Can you work these out from the model? Positions are in its coordinate system, mm. A direction names the side the tool comes from. Coordinates: 2 decimals unless noted, no trailing zeros. Order: outer loops, then holes, each group sorted by start corner. A loop starts at its lowest first (then second) coordinate and runs counter-clockwise, first axis right, second up.
```python
from build123d import *

# Parameters (mm, degrees)
F0_W      = 3.8989
F0_H      = 3.9624
F1_DEPTH  = 3.175
F3_DEPTH  = 38.1
F5_DEPTH  = 64.262
F7_DEPTH  = 63.5
F9_DEPTH  = 25.4
F10_W     = 76.2
F10_H     = 2.617364
F11_DEPTH = 25.4


with BuildPart() as f1:
    # F0 (on Top) → F1 (new body)
    with BuildSketch(Plane.XY):
        Polygon((38.1, 27.7876), (38.1, 31.75), (-34.2011, 31.75), (-34.2011, 27.7876), (-29.4386, 27.7876), (-21.5011, 27.7876), (-16.7386, 27.7876), (-8.6614, 27.7876), (-3.8989, 27.7876), (-3.884394, 27.7876), (4.0386, 27.7876), (8.789393, 27.7876), (8.8011, 27.7876), (16.7386, 27.7876), (21.459464, 27.7876), (21.5011, 27.7876), (29.4386, 27.7876), (34.2011, 27.7876), (34.226403, 27.7876), align=None)
        with Locations((-36.15055, 29.7688)):
            Rectangle(F0_W, F0_H)
        Polygon((38.1, -31.75), (38.1, 27.7876), (34.226403, 27.7876), (34.226403, 23.0251), (29.4386, 23.0251), (29.4386, 27.7876), (21.5011, 27.7876), (21.459464, 27.7876), (21.459464, 23.0251), (16.7386, 23.0251), (16.7386, 27.7876), (8.8011, 27.7876), (8.789393, 27.7876), (8.789393, 23.0251), (4.0386, 23.0251), (4.0386, 27.7876), (-3.884394, 27.7876), (-3.884394, 23.0251), (-8.6614, 23.0251), (-8.6614, 27.7876), (-16.7386, 27.7876), (-16.7386, 23.0251), (-21.5011, 23.0251), (-21.5011, 27.7876), (-29.4386, 27.7876), (-29.4386, 23.0251), (-34.2011, 23.0251), (-34.2011, 15.0876), (-34.2011, 10.3251), (-34.2011, 2.3876), (-34.2011, -2.3749), (-34.2011, -10.3124), (-34.2011, -15.0749), (-34.2011, -23.0124), (-34.2011, -27.7749), (-34.2011, -31.75), align=None)
        Polygon((-34.2011, 23.0251), (-34.2011, 27.7876), (-38.1, 27.7876), (-38.1, -31.75), (-34.2011, -31.75), (-34.2011, -27.7749), (-34.2011, -23.0124), (-34.2011, -15.0749), (-34.2011, -10.3124), (-34.2011, -2.3749), (-34.2011, 2.3876), (-34.2011, 10.3251), (-34.2011, 15.0876), align=None)
    extrude(amount=F1_DEPTH)

    # F2 (on face) → F3 (join)
    with BuildSketch(Plane.XY.offset(3.175)):
        Polygon((-31.75, -28.575), (-31.75, -31.75), (31.75, -31.75), (31.75, -28.575), (31.75, -25.4), (-31.75, -25.4), align=None)
    extrude(amount=F3_DEPTH)

    # F4 (on face) → F5 (cut)
    with BuildSketch(Plane(origin=(-31.75, 0, 0), x_dir=(0, -1, 0), z_dir=(-1, 0, 0))):
        Polygon((31.75, 41.275), (28.575, 41.275), (31.75, 3.175), align=None)
    extrude(amount=-F5_DEPTH, mode=Mode.SUBTRACT)

    # F6 (on face) → F7 (cut)
    with BuildSketch(Plane.YZ.offset(31.75)):
        Polygon((-31.75, 3.175), (-28.575, 3.175), (-26.9875, 41.275), (-28.575, 41.275), align=None)
    extrude(amount=-F7_DEPTH, mode=Mode.SUBTRACT)

    # F8 (on face) → F9 (cut)
    with BuildSketch(Plane.XY.offset(3.175)):
        Polygon((38.1, -28.575), (-31.75, -28.575), (-38.1, -28.575), (-38.1, -31.75), (38.1, -31.75), align=None)
    extrude(amount=-F9_DEPTH, mode=Mode.SUBTRACT)

    # F10 (on face) → F11 (cut)
    with BuildSketch(Plane.XY.offset(3.175)):
        with Locations((0, 30.441318)):
            Rectangle(F10_W, F10_H)
    extrude(amount=-F11_DEPTH, mode=Mode.SUBTRACT)


solid = f1.part
```
1. On a 3-axis mill with a long thin cutter (end or side, diameter ignored), from which of +Z, -Z, +X, -X, +Y, -Y can I reach the whole of each face in a straight line? I mean faces 5 (the flat face through (-19, 27.788, 2)), 6 (the flat face through (31.75, -27, 22)), 7 (the flat face through (-38.1, 1, 2)). Say none if no direction works.
Completed:
face 5: +Z, -Z
face 6: +Z, +X, +Y, -Y
face 7: +Z, -Z, -X, +Y, -Y
2. Imagine slicing it at A-A on x = 6. Please give me the cut outline in (y, z) (1 decimal).
Completed:
outline: (-28.6, 0) - (23, 0) - (23, 3.2) - (-25.4, 3.2) - (-25.4, 41.3) - (-27, 41.3) - (-28.6, 3.2) - close; (27.8, 0) - (29.1, 0) - (29.1, 3.2) - (27.8, 3.2) - close
3. Imagine slicing it at D-D on z = 15. Please give me the cut outline in (x, y).
Completed:
outline: (-31.75, -28.08) - (31.75, -28.08) - (31.75, -25.4) - (-31.75, -25.4) - close
4. I'm going to push flat-ended pins straight in: pin 1 (1.6 mm diameter, centred on y = -27.5, z = 18.5, fed in from -X); pin 2 (1.5 mm diameter, centred on x = -17.5, y = 11.5, fed in from +Z) (3 decimals). Where does each tip first touch, or does it pass through?
Completed:
pin 1: stops at x = -31.75
pin 2: stops at z = 3.175
5. Imagine slicing it at B-B on x = -25. Please give me the cut outline in (y, z) (1 decimal), then the cut area to 3 significant figures.
Completed:
outline: (-28.6, 0) - (29.1, 0) - (29.1, 3.2) - (-25.4, 3.2) - (-25.4, 41.3) - (-27, 41.3) - (-28.6, 3.2) - close
area: 274 mm2
6. Please list where these lines run through material, in increasing order: probe 1 along Z at (x, y) = (-27.5, -16) (3 decimals); probe 2 along Y at (x, z) = (-23, 3.5); probe 3 along Y at (x, z) = (-6.5, 18.5).
Completed:
probe 1: z = 0 to 3.175
probe 2: y = -28.56 to -25.4
probe 3: y = -27.94 to -25.4
7. Thinking about a two-plate mould opening in Y: for faces 1 (the flat face through (0.444, -27.792, 21.958)), 2 (the flat face through (-31.75, -27, 22)), 3 (the flat face through (4.039, 25, 2)), 4 (the flat face through (-1, 29.133, 2)), which applies, pulls with the +Y half, pulls with the -Y half, needs draft (parallel to the pull), parting line crosses it, or undercut?
Completed:
face 1: pulls with the -Y half
face 2: needs draft
face 3: undercut
face 4: pulls with the +Y half
8. Imagine slicing it at C-C on y = -15.5. Please give me the cut outline in (x, z) (3 decimals).
Completed:
outline: (-38.1, 0) - (38.1, 0) - (38.1, 3.175) - (-38.1, 3.175) - close
